Source: CAD feature listing. Evaluate the final solid. Frame: model axes, mm. Face numbers are marked on the shaded views. Give positions to 0.01 mm unless a question says otherwise; leave off trailing zeros. Loops run counter-clockwise (first coordinate to the right, second up) from the corner with the lowest first, then second, coordinate; pieces in that order, holes last. Notation, with made-up numbers: (80.5, -3) -> (101.5, -3) arc R6 ccw to (101.5, 4) -> close; hole circle Ø2 at (26, 15). An arc over 180 degrees is marked (long way). Answer as a JSON object with one key per item and string values. Group by question number.
from build123d import *

# Parameters (mm, degrees)
CROQUIS1_W              = 74
CROQUIS1_H              = 128
SALIENTE_EXTRUIR1_DEPTH = 11.5
CROQUIS2_W              = 80
CROQUIS2_H              = 154
CORTAR_EXTRUIR1_DEPTH   = 10.5
SALIENTE_EXTRUIR3_DEPTH = 154


with BuildPart() as part:
    # Croquis1 → Saliente-Extruir1 (new body)
    with BuildSketch(Plane.XY):
        Polygon((-40, 77), (-41.5, 77), (-41.5, -78.5), (41.5, -78.5), (41.5, 77), (40, 77), align=None)
        with Locations((0, 3)):
            Rectangle(CROQUIS1_W, CROQUIS1_H, mode=Mode.SUBTRACT)
    extrude(amount=SALIENTE_EXTRUIR1_DEPTH)

    # Croquis2 → Cortar-Extruir1 (cut)
    with BuildSketch(Plane(origin=(0, 0, 0), x_dir=(-1, 0, 0), z_dir=(0, 0, -1))):
        Rectangle(CROQUIS2_W, CROQUIS2_H)
    extrude(amount=-CORTAR_EXTRUIR1_DEPTH, mode=Mode.SUBTRACT)

    # Croquis3 → Saliente-Extruir3 (add, through all)
    with BuildSketch(Plane(origin=(0, -77, 0), x_dir=(1, 0, 0), z_dir=(0, 1, 0))):
        Polygon((-40, -5.5), (-35, 0), (-40, 0), align=None)
        Polygon((40, 0), (40, -5.5), (35, 0), align=None)
    extrude(amount=SALIENTE_EXTRUIR3_DEPTH)


solid = part.part
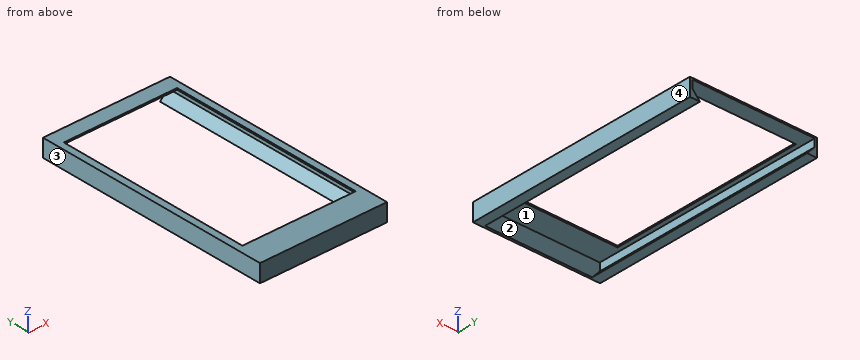
(1) Mould query, pull axis X, two halves, no side actions, for the marked faces 1, 2, 3 and 4. Classes: pulls with the +X half, pulls with the -X half, needs draft (parallel to the pull), parting line crosses it, or undercut.
(2) Section query A-A on y = 52.5. Return the cut outline in (x, z), plus the area to 3 significant figures.
(3) Material intervals for line 1 (X direction, y = -46.5, z = 10); line 2 (X direction, y = 10.5, z = 10.75); line 3 (Y direction, x = -20, z = 1), sorted ascending. Write a range as from..to.
(4) Section query C-C on z = 7. Return the cut outline in (x, y), plus the area to 4 significant figures.
(5) First-contact query: pin 1 (5 mm diameter, centred on x = -6.5, z = 7.5, fed in from +Y). Flat tip, straight axial feed; report the tip coordinate or a pass-through.
(6) Section query B-B on x = -13. Return the cut outline in (y, z).
Result:
{
 "1": {"face 1": "undercut", "face 2": "undercut", "face 3": "pulls with the -X half", "face 4": "pulls with the +X half"},
 "2": {"outline": "(-41.5, 0) -> (-35, 0) -> (-40, 5.5) -> (-40, 10.5) -> (-37, 10.5) -> (-37, 11.5) -> (-41.5, 11.5) -> close; (35, 0) -> (41.5, 0) -> (41.5, 11.5) -> (37, 11.5) -> (37, 10.5) -> (40, 10.5) -> (40, 5.5) -> close", "area": "68.0 mm²"},
 "3": {"line 1": "-41.5..-40, 40..41.5", "line 2": "-41.5..-37, 37..41.5", "line 3": "-78.5..-77"},
 "4": {"outline": "(-41.5, -78.5) -> (41.5, -78.5) -> (41.5, 77) -> (40, 77) -> (40, -77) -> (-40, -77) -> (-40, 77) -> (-41.5, 77) -> close", "area": "586.5 mm²"},
 "5": {"pin 1": "y = -77"},
 "6": {"outline": "(-78.5, 0) -> (-77, 0) -> (-77, 10.5) -> (-61, 10.5) -> (-61, 11.5) -> (-78.5, 11.5) -> close; (67, 10.5) -> (77, 10.5) -> (77, 11.5) -> (67, 11.5) -> close"}
}
